```python
from build123d import *

# Parameters (mm, degrees)
SKETCH1_W           = 112
SKETCH1_H           = 64
BOSS_EXTRUDE1_DEPTH = 16
SKETCH3_W           = 16
SKETCH3_H           = 40
BOSS_EXTRUDE2_DEPTH = 32
SKETCH6_W           = 16
SKETCH6_H           = 40
BOSS_EXTRUDE3_DEPTH = 32
CUT_EXTRUDE1_REACH  = 133.21
SKETCH7_W           = 32
SKETCH7_H           = 24


with BuildPart() as part:
    # Sketch1 → Boss-Extrude1 (new body)
    with BuildSketch(Plane(origin=(0, 0, 0), x_dir=(1, 0, 0), z_dir=(0, 1, 0))):
        with Locations((56, 32)):
            Rectangle(SKETCH1_W, SKETCH1_H)
    extrude(amount=BOSS_EXTRUDE1_DEPTH)

    # Sketch3 → Boss-Extrude2 (add)
    with BuildSketch(Plane.XY):
        with Locations((8, 20)):
            Rectangle(SKETCH3_W, SKETCH3_H)
    extrude(amount=-BOSS_EXTRUDE2_DEPTH)

    # Sketch6 → Boss-Extrude3 (add)
    with BuildSketch(Plane(origin=(0, 0, -64), x_dir=(-1, 0, 0), z_dir=(0, 0, -1))):
        with Locations((-104, 20)):
            Rectangle(SKETCH6_W, SKETCH6_H)
    extrude(amount=-BOSS_EXTRUDE3_DEPTH)

    # Sketch7 → Cut-Extrude1 (cut, up to next)
    with BuildSketch(Plane(origin=(0, 16, 0), x_dir=(1, 0, 0), z_dir=(0, 1, 0)), mode=Mode.PRIVATE) as cut_extrude1_sk1:
        with Locations((56, 32)):
            Rectangle(SKETCH7_W, SKETCH7_H)
    cut_extrude1_tool1 = extrude(cut_extrude1_sk1.sketch, amount=-CUT_EXTRUDE1_REACH, mode=Mode.PRIVATE) & part.part
    add(cut_extrude1_tool1.solids().sort_by_distance((56, 16, -32))[0], mode=Mode.SUBTRACT)


solid = part.part
```
Model file for the job. Use its own axes, mm. A direction names the side the tool comes from. Give positions to 0.01 mm unless a question says otherwise; leave off trailing zeros. Write each loop counter-clockwise with the first axis right and the second up, starting at its lowest first coordinate (ties: lowest second). Pieces come first, ordered by that corner, then holes. Notation, with made-up numbers: M -16,68.25 L 19,68.25 A9 ccw 19,85.25 Z; hole C 6.25,77 d5. An arc over 180 degrees is marked long. Use a Markdown table: item, result.
1) Cut at C-C (y = 12.5). List the corners of the cut face in (x, z).
Responses:
| item | result |
|---|---|
| outline | M 0,-64 L 112,-64 L 112,0 L 0,0 Z; hole M 40,-44 L 72,-44 L 72,-20 L 40,-20 Z |
2) Cut at B-B (x = 56). List the corners of the cut face in (y, z).
Responses:
| item | result |
|---|---|
| outline | M 0,-64 L 16,-64 L 16,-44 L 0,-44 Z; M 0,-20 L 16,-20 L 16,0 L 0,0 Z |
3) Tool access for faces 1 (the flat face through (104, 28, -32)), 2 (the flat face through (8, 28, -32)), 3 (the flat face through (16, 28, -16)), 4 (the flat face through (72, 8, -32)): list every direction of +Z, -Z, +X, -X, +Y, -Y with a clear straight run to the whole face (end or side of a thin tool).
Responses:
| item | result |
|---|---|
| face 1 | +Z, +X, +Y |
| face 2 | -Z, -X, +Y |
| face 3 | +Z, -Z, +X, +Y |
| face 4 | +Y, -Y |
4) Drill centre lines: line 1 (X direction, y = 10.5, z = -37.5); line 2 (Z direction, x = 66.5, y = 6.5); line 3 (X direction, y = 23.5, z = -51). Where is each one in solid material? Low to high. Write a range as from..to.
Responses:
| item | result |
|---|---|
| line 1 | x = 0..40, 72..112 |
| line 2 | z = -64..-44, -20..0 |
| line 3 | x = 96..112 |
5) Pin check, flat tips, straight feed: pin 1 (7 mm diameter, centred on y = 26.5, z = -13.5, fed in from +X); pin 2 (6 mm diameter, centred on y = 26.5, z = -52, fed in from -X); pin 3 (19 mm diameter, centred on x = 82, z = -16.5, fed in from +Y). Stop position of each tip, or through.
Responses:
| item | result |
|---|---|
| pin 1 | stops at x = 16 |
| pin 2 | stops at x = 96 |
| pin 3 | stops at y = 16 |
6) Cut at D-D (y = 35.5). List the corners of the cut face in (x, z).
Responses:
| item | result |
|---|---|
| outline | M 0,-32 L 16,-32 L 16,0 L 0,0 Z; M 96,-64 L 112,-64 L 112,-32 L 96,-32 Z |
7) Cut at A-A (z = -36). List the corners of the cut face in (x, y), and give its area (3 significant figures).
Responses:
| item | result |
|---|---|
| outline | M 0,0 L 40,0 L 40,16 L 0,16 Z; M 72,0 L 112,0 L 112,40 L 96,40 L 96,16 L 72,16 Z |
| area | 1,660 mm2 |
